```python
from build123d import *

# Parameters (mm, degrees)
BOSS_EXTRUDE1_DEPTH = 6
SKETCH4_W           = 44.8
SKETCH4_H           = 34.8
SKETCH4_R           = 1.5
BOSS_EXTRUDE3_DEPTH = 2
FILLET1_R           = 2
CHAMFER1_SIZE       = 0.75
SKETCH5_R           = 4.5
CUT_EXTRUDE1_DEPTH  = 29.991722957


with BuildPart() as part:
    # Sketch1 → Boss-Extrude1 (new body)
    with BuildSketch(Plane.YZ):
        with BuildLine():
            Line((-12.197438256, -0.25), (-11.197209474, -0.25))
            ThreePointArc((-11.197209474, -0.25), (11.2, 0), (-11.197209474, 0.25))
            Line((-11.197209474, 0.25), (-12.197438256, 0.25))
            ThreePointArc((-12.197438256, 0.25), (12.2, 0), (-12.197438256, -0.25))
        make_face()
    extrude(amount=BOSS_EXTRUDE1_DEPTH)

    # Sketch4 → Boss-Extrude3 (add)
    with BuildSketch(Plane(origin=(0, 0, 0), x_dir=(0, -1, 0), z_dir=(-1, 0, 0))):
        Rectangle(SKETCH4_W, SKETCH4_H)
        with Locations(Location((-18.9, 13.9, 0), (0, 0, 90))):
            Circle(SKETCH4_R, mode=Mode.SUBTRACT)
        with Locations(Location((18.9, 13.9, 0), (0, 0, 90))):
            Circle(SKETCH4_R, mode=Mode.SUBTRACT)
        with Locations(Location((-18.9, -13.9, 0), (0, 0, 90))):
            Circle(SKETCH4_R, mode=Mode.SUBTRACT)
        with Locations(Location((18.9, -13.9, 0), (0, 0, 90))):
            Circle(SKETCH4_R, mode=Mode.SUBTRACT)
    extrude(amount=BOSS_EXTRUDE3_DEPTH)

    # Fillet1
    fillet1_edges = [part.edges().sort_by_distance(p)[0] for p in [
        (-1, -22.4, 17.4),
        (-1, 22.4, 17.4),
        (-1, 22.4, -17.4),
        (-1, -22.4, -17.4),
    ]]
    fillet(fillet1_edges, radius=FILLET1_R)

    # Chamfer1
    chamfer1_edges = [part.edges().sort_by_distance(p)[0] for p in [
        (6, 11.2, 0),
    ]]
    chamfer(chamfer1_edges, length=CHAMFER1_SIZE)

    # Sketch5 → Cut-Extrude1 (cut, through all)
    with BuildSketch(Plane.YZ):
        with Locations(Location((0, 0, 0), (0, 0, 270))):
            Circle(SKETCH5_R)
    extrude(amount=-CUT_EXTRUDE1_DEPTH, mode=Mode.SUBTRACT)


solid = part.part
```
The model under review builds one solid part; all positions refer to its coordinate system, in mm. A direction names the side the tool comes from. Round coordinates to 2 decimals unless told otherwise and drop trailing zeros. Write each loop counter-clockwise with the first axis right and the second up, starting at its lowest first coordinate (ties: lowest second). Pieces come first, ordered by that corner, then holes. Notation, with made-up numbers: (41, -40) - (62, -40) arc R24 cw to (62, -3) - close; hole circle Ø1 at (86, -8). An arc over 180 degrees is marked (long way). Answer as CSV lines item,"result". Start each with the question number.
(1) Draft analysis for pull direction Z (two halves, no side actions). For faces 1 (the flat face through (3, -12, -0.25)), 2 (the flat face through (-1, 22.4, 0)), 3 (the cylindrical face through (-1.01, 21.83, 16.8)), state which applies: pulls with the +Z half, pulls with the -Z half, needs draft (parallel to the pull), parting line crosses it, or undercut.
(2) To check wall thickness, follow line 1 (Y direction, x = -1.4, z = 13.9); line 2 (Y direction, x = 4.25, z = 0.5). State the ranges of each line that lie inside material, in increasing order.
(3) We need section B-B on z = -13.9. State the section outline as (x, y) points, plus the area to 3 significant figures.
(4) We need section C-C on y = 0. State the section outline as (x, z) points, plus the area to 3 significant figures.
(5) For faces 4 (the flat face through (0, 5, 0)), 5 (the flat face through (3, -12, 0.25)), 6 (the cylindrical face through (-0.986, 1.352, -4.292)), list the 3-axis set-ups (+Z, -Z, +X, -X, +Y, -Y) from which the entire face can be reached by the end or side of a thin tool; tool diameter is ignored.
(6) For pin 1 Ø3.5 at (y, z) = (-18.9, -13.9) entering from +X; pin 2 Ø3 at (x, z) = (5, -12.5) entering from -Y; pin 3 Ø18 at (y, z) = (0, 0) entering from -X; pin 4 Ø7 at (y, z) = (0, 0) entering from -X, all flat-tipped, find the tip position at first contact; note any pin that passes through.
(7) We need section A-A on y = -18.9. State the section outline as (x, z) points.
(8) We need section D-D on x = 3.25. State the section outline as (y, z) points.
Worked answers:
1,face 1,"undercut"
1,face 2,"needs draft"
1,face 3,"pulls with the +Z half"
2,line 1,"-22.4 to -20.4, -17.4 to 17.4, 20.4 to 22.4"
2,line 2,"-12.19 to -11.19, 11.19 to 12.19"
3,outline,"(-2, -22.4) - (0, -22.4) - (0, -20.4) - (-2, -20.4) - close; (-2, -17.4) - (0, -17.4) - (0, 17.4) - (-2, 17.4) - close; (-2, 20.4) - (0, 20.4) - (0, 22.4) - (-2, 22.4) - close"
3,area,"77.6 mm²"
4,outline,"(-2, -17.4) - (0, -17.4) - (0, -12.2) - (6, -12.2) - (6, -11.95) - (5.25, -11.2) - (0, -11.2) - (0, -4.5) - (-2, -4.5) - close; (-2, 4.5) - (0, 4.5) - (0, 11.2) - (5.25, 11.2) - (6, 11.95) - (6, 12.2) - (0, 12.2) - (0, 17.4) - (-2, 17.4) - close"
4,area,"63.0 mm²"
5,face 4,"+X"
5,face 5,"+X, -Y"
5,face 6,"+X, -X"
6,pin 1,"x = 0"
6,pin 2,"y = -5.28"
6,pin 3,"x = -2"
6,pin 4,"through"
7,outline,"(-2, -17.4) - (0, -17.4) - (0, -15.4) - (-2, -15.4) - close; (-2, -12.4) - (0, -12.4) - (0, 12.4) - (-2, 12.4) - close; (-2, 15.4) - (0, 15.4) - (0, 17.4) - (-2, 17.4) - close"
8,outline,"(-12.2, -0.25) arc R12.2 ccw (long way) to (-12.2, 0.25) - (-11.2, 0.25) arc R11.2 cw (long way) to (-11.2, -0.25) - close"
